Build history of the part. All positions in model axes, mm. A direction names the side the tool comes from. Round coordinates to 2 decimals unless told otherwise and drop trailing zeros. Loops run counter-clockwise (first coordinate to the right, second up) from the corner with the lowest first, then second, coordinate; pieces in that order, holes last.
from build123d import *

# Parameters (mm, degrees)
SKETCH1_R           = 7.25
BOSS_EXTRUDE1_DEPTH = 5.8
SKETCH2_R           = 6.325
CUT_EXTRUDE1_DEPTH  = 1.5875
SKETCH3_R           = 1
BOSS_EXTRUDE2_DEPTH = 1.5875
SKETCH4_R           = 3.15
BOSS_EXTRUDE3_DEPTH = 3
SKETCH5_R           = 0.85
CUT_EXTRUDE2_DEPTH  = 38.866125059
SKETCH6_R           = 1.11
CUT_EXTRUDE3_DEPTH  = 3


with BuildPart() as part:
    # Sketch1 → Boss-Extrude1 (new body)
    with BuildSketch(Plane.XY):
        with Locations((-29.082250471, -1.703826149)):
            Circle(SKETCH1_R)
    extrude(amount=BOSS_EXTRUDE1_DEPTH)

    # Sketch2 → Cut-Extrude1 (cut)
    with BuildSketch(Plane(origin=(0, 0, 0), x_dir=(-1, 0, 0), z_dir=(0, 0, -1))):
        with Locations((29.082250471, -1.703826149)):
            Circle(SKETCH2_R)
    extrude(amount=-CUT_EXTRUDE1_DEPTH, mode=Mode.SUBTRACT)

    # Sketch3 → Boss-Extrude2 (add)
    with BuildSketch(Plane(origin=(0, 0, 1.5875), x_dir=(-1, 0, 0), z_dir=(0, 0, -1))):
        with Locations((29.082250471, -1.703826149)):
            Circle(SKETCH3_R)
    extrude(amount=BOSS_EXTRUDE2_DEPTH)

    # Sketch4 → Boss-Extrude3 (add)
    with BuildSketch(Plane(origin=(0, 0, 0), x_dir=(-1, 0, 0), z_dir=(0, 0, -1))):
        with Locations((29.082250471, -1.703826149)):
            Circle(SKETCH4_R)
    extrude(amount=-BOSS_EXTRUDE3_DEPTH)

    # Sketch5 → Cut-Extrude2 (cut, through all)
    with BuildSketch(Plane(origin=(0, 0, 0), x_dir=(-1, 0, 0), z_dir=(0, 0, -1))):
        with Locations((29.082250471, -1.703826149)):
            Circle(SKETCH5_R)
    extrude(amount=-CUT_EXTRUDE2_DEPTH, mode=Mode.SUBTRACT)

    # Sketch6 → Cut-Extrude3 (cut)
    with BuildSketch(Plane.XY.offset(5.8)):
        with Locations((-29.082250471, -1.703826149)):
            Circle(SKETCH6_R)
    extrude(amount=-CUT_EXTRUDE3_DEPTH, mode=Mode.SUBTRACT)


solid = part.part
(1) Slice it at A-A on x = -29. List the corners of the cut face in (y, z).
Responses:
outline: (-8.95, 0) - (-8.03, 0) - (-8.03, 1.59) - (-4.85, 1.59) - (-4.85, 0) - (-2.55, 0) - (-2.55, 2.8) - (-2.81, 2.8) - (-2.81, 5.8) - (-8.95, 5.8) - close; (-0.86, 0) - (1.45, 0) - (1.45, 1.59) - (4.62, 1.59) - (4.62, 0) - (5.55, 0) - (5.55, 5.8) - (-0.6, 5.8) - (-0.6, 2.8) - (-0.86, 2.8) - close
(2) Which spindle directions (+Z, -Z, +X, -X, +Y, -Y) get a long thin tool onto all of the face, cutting with end or side? Do faces 1 (the face through (-30.19, -1.66, 4.32)), 2 (the face through (-30, -1, 0)), 3 (the face through (-35.115, 0.196, 0.783)). Say none if no direction does.
Responses:
face 1: +Z
face 2: -Z, +X, -X, +Y, -Y
face 3: -Z
(3) Probe line 1 (Y direction, x = -29, z = 0.5); line 2 (X direction, y = -3.5, z = 1.35); line 3 (X direction, y = -4, z = 1.35). List the from-to ranges inside material, lowest first.
Responses:
line 1: y = -8.95 to -8.03, -4.85 to -2.55, -0.86 to 1.45, 4.62 to 5.55
line 2: x = -36.11 to -35.15, -31.67 to -26.49, -23.02 to -22.06
line 3: x = -35.96 to -34.98, -31.24 to -26.93, -23.19 to -22.21
(4) Slice it at D-D on x = -31. List the corners of the cut face in (y, z).
Responses:
outline: (-8.7, 0) - (-7.73, 0) - (-7.73, 1.59) - (-4.2, 1.59) - (-4.2, 0) - (0.8, 0) - (0.8, 1.59) - (4.32, 1.59) - (4.32, 0) - (5.29, 0) - (5.29, 5.8) - (-8.7, 5.8) - close
(5) Slice it at C-C on z = 0.55. List the corners of the cut face in (x, y) (3 decimals).
Responses:
outline: circle Ø14.5 at (-29.082, -1.704); circle Ø6.3 at (-29.082, -1.704); hole circle Ø12.65 at (-29.082, -1.704); hole circle Ø1.7 at (-29.082, -1.704)
(6) Pin check, flat tips, straight feed: P1, Ø2, axis at x = -29.08, y = -1.7, coming from the +Z side; P2, Ø3, axis at y = 4, z = 3.5, coming from the -X side. Stop position of each tip, or through.
Responses:
P1: stops at z = 2.8
P2: stops at x = -34.99
(7) Pull direction X, two halves, no side cores. Call faces 4 (the face through (-29, -3, 5.8)), 5 (the face through (-31.992, -2.91, 0.783)), 6 (the face through (-22.385, -4.481, 2.859)): +X half, -X half, draft (parallel to the pull), parting line (faces both ways), or undercut.
Responses:
face 4: draft
face 5: undercut
face 6: parting line
(8) Slice it at B-B on y = -1.25. List the corners of the cut face in (x, z).
Responses:
outline: (-36.32, 0) - (-35.39, 0) - (-35.39, 1.59) - (-32.2, 1.59) - (-32.2, 0) - (-29.8, 0) - (-29.8, 2.8) - (-30.1, 2.8) - (-30.1, 5.8) - (-36.32, 5.8) - close; (-28.36, 0) - (-25.97, 0) - (-25.97, 1.59) - (-22.77, 1.59) - (-22.77, 0) - (-21.85, 0) - (-21.85, 5.8) - (-28.07, 5.8) - (-28.07, 2.8) - (-28.36, 2.8) - close
